```python
from build123d import *

# Parameters (mm, degrees)
SKETCH_1_W                        = 208
SKETCH_1_H                        = 80
SM_BASE_FLANGE_1_DEPTH            = 2
SM_EDGE_FLANGE_1_STRIP_W          = 9
SM_EDGE_FLANGE_1_STRIP_H          = 2
SM_EDGE_FLANGE_1_STRIP_CUT_DEPTH  = 148
SM_EDGE_FLANGE_1_RELIEF_W         = 10
SM_EDGE_FLANGE_1_RELIEF_H         = 1
SM_EDGE_FLANGE_1_RELIEF_CUT_DEPTH = 2
SM_EDGE_FLANGE_1_DEPTH            = 148
SM_EDGE_FLANGE_2_STRIP_W          = 9
SM_EDGE_FLANGE_2_STRIP_H          = 2
SM_EDGE_FLANGE_2_STRIP_CUT_DEPTH  = 148
SM_EDGE_FLANGE_2_RELIEF_W         = 10
SM_EDGE_FLANGE_2_RELIEF_H         = 1
SM_EDGE_FLANGE_2_RELIEF_CUT_DEPTH = 2
SM_EDGE_FLANGE_2_DEPTH            = 148
SKETCH_10_R                       = 3.5
CUT_EXTRUDE_1_DEPTH               = 114.207773585
FILLET_1_R                        = 3


# Sheet-metal steps are written as plain solids
with BuildPart() as part:
    # Sketch 1 → 基体-法兰1 (new body)
    with BuildSketch(Plane.XY):
        Rectangle(SKETCH_1_W, SKETCH_1_H)
    extrude(amount=-SM_BASE_FLANGE_1_DEPTH)

    # 边线-法兰1 strip (across the edge) → 边线-法兰1 strip cut (cut)
    with BuildSketch(Plane(origin=(-74, 40, -2), x_dir=(0, -1, 0), z_dir=(1, 0, 0))):
        with Locations((-2, -1)):
            Rectangle(SM_EDGE_FLANGE_1_STRIP_W, SM_EDGE_FLANGE_1_STRIP_H)
    extrude(amount=SM_EDGE_FLANGE_1_STRIP_CUT_DEPTH, mode=Mode.SUBTRACT)

    # 边线-法兰1 relief (on the sheet) → 边线-法兰1 relief cut (cut)
    with BuildSketch(Plane(origin=(-74, 37.5, -2), x_dir=(0, -1, 0), z_dir=(0, 0, -1))):
        with Locations((-4, 0.5)):
            Rectangle(SM_EDGE_FLANGE_1_RELIEF_W, SM_EDGE_FLANGE_1_RELIEF_H)
        with Locations((-4, -148.5)):
            Rectangle(SM_EDGE_FLANGE_1_RELIEF_W, SM_EDGE_FLANGE_1_RELIEF_H)
    extrude(amount=-SM_EDGE_FLANGE_1_RELIEF_CUT_DEPTH, mode=Mode.SUBTRACT)

    # 边线-法兰1 section (across the edge) → 边线-法兰1 (add)
    with BuildSketch(Plane(origin=(-74, 40, -2), x_dir=(0, -1, 0), z_dir=(1, 0, 0))):
        with BuildLine():
            Line((0, 0.5), (0, 18))
            Line((0, 18), (2, 18))
            Line((2, 18), (2, 0.5))
            ThreePointArc((2, 0.5), (2.146446609, 0.146446609), (2.5, 0))
            Line((2.5, 0), (2.5, -2))
            ThreePointArc((2.5, -2), (0.732233047, -1.267766953), (0, 0.5))
        make_face()
    extrude(amount=SM_EDGE_FLANGE_1_DEPTH)

    # 边线-法兰2 strip (across the edge) → 边线-法兰2 strip cut (cut)
    with BuildSketch(Plane(origin=(74, -40, -2), x_dir=(0, 1, 0), z_dir=(-1, 0, 0))):
        with Locations((-2, -1)):
            Rectangle(SM_EDGE_FLANGE_2_STRIP_W, SM_EDGE_FLANGE_2_STRIP_H)
    extrude(amount=SM_EDGE_FLANGE_2_STRIP_CUT_DEPTH, mode=Mode.SUBTRACT)

    # 边线-法兰2 relief (on the sheet) → 边线-法兰2 relief cut (cut)
    with BuildSketch(Plane(origin=(74, -37.5, -2), x_dir=(0, 1, 0), z_dir=(0, 0, -1))):
        with Locations((-4, 0.5)):
            Rectangle(SM_EDGE_FLANGE_2_RELIEF_W, SM_EDGE_FLANGE_2_RELIEF_H)
        with Locations((-4, -148.5)):
            Rectangle(SM_EDGE_FLANGE_2_RELIEF_W, SM_EDGE_FLANGE_2_RELIEF_H)
    extrude(amount=-SM_EDGE_FLANGE_2_RELIEF_CUT_DEPTH, mode=Mode.SUBTRACT)

    # 边线-法兰2 section (across the edge) → 边线-法兰2 (add)
    with BuildSketch(Plane(origin=(74, -40, -2), x_dir=(0, 1, 0), z_dir=(-1, 0, 0))):
        with BuildLine():
            Line((0, 0.5), (0, 18))
            Line((0, 18), (2, 18))
            Line((2, 18), (2, 0.5))
            ThreePointArc((2, 0.5), (2.146446609, 0.146446609), (2.5, 0))
            Line((2.5, 0), (2.5, -2))
            ThreePointArc((2.5, -2), (0.732233047, -1.267766953), (0, 0.5))
        make_face()
    extrude(amount=SM_EDGE_FLANGE_2_DEPTH)

    # 草图10 → 切除-拉伸1 (cut, through all)
    with BuildSketch(Plane.XY):
        with Locations((91, -30)):
            Circle(SKETCH_10_R)
        with Locations((91, 30)):
            Circle(SKETCH_10_R)
        with Locations((-91, -30)):
            Circle(SKETCH_10_R)
        with Locations((-91, 30)):
            Circle(SKETCH_10_R)
    extrude(amount=-CUT_EXTRUDE_1_DEPTH, mode=Mode.SUBTRACT)

    # 圆角1
    fillet_1_edges = [part.edges().sort_by_distance(p)[0] for p in [
        (-74, 39, -20),
        (74, 39, -20),
        (104, -40, -1),
        (-104, -40, -1),
        (-104, 40, -1),
        (104, 40, -1),
        (74, -39, -20),
        (-74, -39, -20),
    ]]
    fillet(fillet_1_edges, radius=FILLET_1_R)


solid = part.part
```
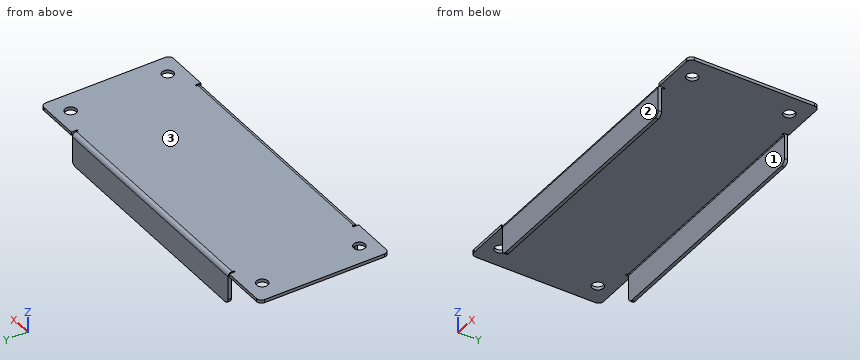
Geometry check sheet. Reference: the model listing, model coordinates, mm. Face numbers are marked on the shaded views. Round coordinates to 2 decimals unless told otherwise and drop trailing zeros. Loops run counter-clockwise (first coordinate to the right, second up) from the corner with the lowest first, then second, coordinate; pieces in that order, holes last. Notation, with made-up numbers: (72.5, 13.25) - (108.5, 13.25) arc R18 cw to (108.5, 33.25) - close; hole circle Ø11 at (5, 65). An arc over 180 degrees is marked (long way). Use a Markdown table: item, result.
Q1. Go/stop test with flat-tipped pins: P1, Ø1.8, axis at y = 38.5, z = -6, coming from the +X side; P2, Ø8, axis at x = -91, y = -30, coming from the -Z side; P3, Ø4, axis at y = 39, z = -7, coming from the -X side; P4, Ø3, axis at x = 9, y = -8.5, coming from the +Z side. Record where each tip stops, or that it passes through.
Solutions:
| item | result |
|---|---|
| P1 | stops at x = 74 |
| P2 | stops at z = -2 |
| P3 | stops at x = -74 |
| P4 | stops at z = 0 |
Q2. Material ranges on line 1 (Y direction, x = 91, z = -0.65); line 2 (Y direction, x = -20, z = -18); line 3 (Z direction, x = 19.5, y = 27.5), recorded low to high.
Solutions:
| item | result |
|---|---|
| line 1 | y = -40 to -33.5, -26.5 to 26.5, 33.5 to 40 |
| line 2 | y = -40 to -38, 38 to 40 |
| line 3 | z = -2 to 0 |
Q3. Cross-section at A-A on z = -6. Record the cut outline in (x, y).
Solutions:
| item | result |
|---|---|
| outline | (-74, -40) - (74, -40) - (74, -38) - (-74, -38) - close; (-74, 38) - (74, 38) - (74, 40) - (-74, 40) - close |
Q4. Draft check along Y on the marked faces 1, 2 and 3. Enter one of: released by +Y, released by -Y, zero draft, split by the parting line, or undercut.
Solutions:
| item | result |
|---|---|
| face 1 | undercut |
| face 2 | released by -Y |
| face 3 | zero draft |
Q5. Cross-section at B-B on x = -91. Record the cut outline in (y, z).
Solutions:
| item | result |
|---|---|
| outline | (-40, -2) - (-33.5, -2) - (-33.5, 0) - (-40, 0) - close; (-26.5, -2) - (26.5, -2) - (26.5, 0) - (-26.5, 0) - close; (33.5, -2) - (40, -2) - (40, 0) - (33.5, 0) - close |
Q6. Cross-section at D-D on x = -39.5. Record the cut outline in (y, z).
Solutions:
| item | result |
|---|---|
| outline | (-40, -20) - (-38, -20) - (-38, -2.5) arc R0.5 cw to (-37.5, -2) - (37.5, -2) arc R0.5 cw to (38, -2.5) - (38, -20) - (40, -20) - (40, -2.5) arc R2.5 ccw to (37.5, 0) - (-37.5, 0) arc R2.5 ccw to (-40, -2.5) - close |
Q7. Cross-section at C-C on y = -30. Record the cut outline in (x, z), plus the area to 3 significant figures.
Solutions:
| item | result |
|---|---|
| outline | (-104, -2) - (-94.5, -2) - (-94.5, 0) - (-104, 0) - close; (-87.5, -2) - (87.5, -2) - (87.5, 0) - (-87.5, 0) - close; (94.5, -2) - (104, -2) - (104, 0) - (94.5, 0) - close |
| area | 388 mm2 |
